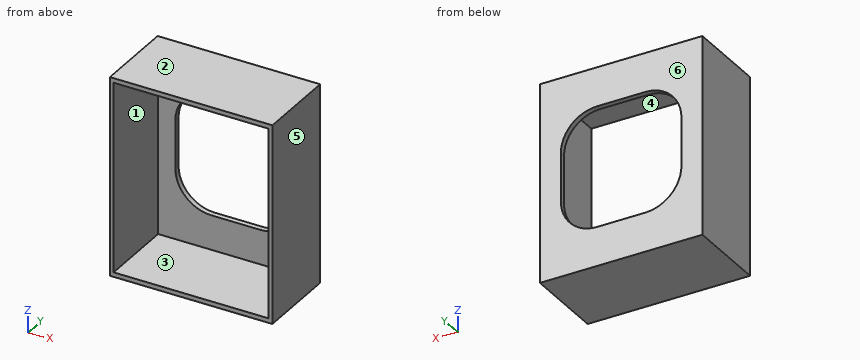
from build123d import *

# Parameters (mm, degrees)
SKETCH1_W           = 90
SKETCH1_H           = 110
BOSS_EXTRUDE1_DEPTH = 3
CUT_EXTRUDE5_DEPTH  = 72.126647608
SKETCH3_W           = 90
SKETCH3_H           = 110
SKETCH3_W_2         = 85.90909091
SKETCH3_H_2         = 105
BOSS_EXTRUDE2_DEPTH = 42


with BuildPart() as part:
    # Sketch1 → Boss-Extrude1 (new body)
    with BuildSketch(Plane(origin=(0, 12.45, 0), x_dir=(1, 0, 0), z_dir=(0, 1, 0))):
        Rectangle(SKETCH1_W, SKETCH1_H)
    extrude(amount=-BOSS_EXTRUDE1_DEPTH)

    # Sketch2 → Cut-Extrude5 (cut, through all)
    with BuildSketch(Plane(origin=(0, 12.45, 0), x_dir=(1, 0, 0), z_dir=(0, 1, 0))):
        with BuildLine():
            Line((-13.4, 33.399999142), (13.4, 33.399999142))
            ThreePointArc((13.4, 33.399999142), (27.542135624, 27.542134765), (33.4, 13.399999142))
            Line((33.4, 13.399999142), (33.4, -13.399999142))
            ThreePointArc((33.4, -13.399999142), (27.542135624, -27.542134765), (13.4, -33.399999142))
            Line((13.4, -33.399999142), (-13.4, -33.399999142))
            ThreePointArc((-13.4, -33.399999142), (-27.542135624, -27.542134765), (-33.4, -13.399999142))
            Line((-33.4, -13.399999142), (-33.4, 13.399999142))
            ThreePointArc((-33.4, 13.399999142), (-27.542135624, 27.542134765), (-13.4, 33.399999142))
        make_face()
    extrude(amount=-CUT_EXTRUDE5_DEPTH, mode=Mode.SUBTRACT)

    # Sketch3 → Boss-Extrude2 (add)
    with BuildSketch(Plane.XZ.offset(-9.45)):
        Rectangle(SKETCH3_W, SKETCH3_H)
        Rectangle(SKETCH3_W_2, SKETCH3_H_2, mode=Mode.SUBTRACT)
    extrude(amount=BOSS_EXTRUDE2_DEPTH)


solid = part.part
Design review of the part built by this model. Coordinates are the model's own, in mm. Face numbers are marked on the shaded views. A direction names the side the tool comes from. Round coordinates to 2 decimals unless told otherwise and drop trailing zeros. Write each loop counter-clockwise with the first axis right and the second up, starting at its lowest first coordinate (ties: lowest second). Pieces come first, ordered by that corner, then holes.
Item 1: For the marked faces 1 and 2, list the 3-axis set-ups (+Z, -Z, +X, -X, +Y, -Y) from which the entire face can be reached by the end or side of a thin tool; tool diameter is ignored.
Item 2: For pin 1 Ø6 at (x, z) = (-33, -20.5) entering from -Y, flat-tipped, find the tip position at first contact; note if it passes through.
Item 3: Wall thickness on L1, parallel to Z at x = 8, y = -9.5; L2, parallel to X at y = -30, z = 47.5; L3, parallel to Y at x = 40.5, z = 13: over which ranges is each line inside the solid? List them lowest first.
Item 4: Consider section D-D on x = 37.5. Give the boundary of the cut face in (y, z), and give its area (3 significant figures).
Item 5: Consider section A-A on x = -19. Give the boundary of the cut face in (y, z), and give its area (3 significant figures).
Item 6: Draft analysis for pull direction X (two halves, no side actions). For the marked faces 3, 4, 5 and 6, state which applies: released by +X, released by -X, zero draft, split by the parting line, or undercut.
Item 7: Consider section C-C on y = -16. Give the boundary of the cut face in (x, z).
Item 8: Consider section B-B on z = -7.5. Give the boundary of the cut face in (x, y).
Check values:
1. face 1: -Y
1. face 2: +Z, +X, -X, +Y, -Y
2. pin 1: stops at y = 9.45
3. L1: z = -55 to -52.5, 52.5 to 55
3. L2: x = -45 to -42.95, 42.95 to 45
3. L3: y = 9.45 to 12.45
4. outline: (-32.55, -55) - (12.45, -55) - (12.45, 55) - (-32.55, 55) - (-32.55, 52.5) - (9.45, 52.5) - (9.45, -52.5) - (-32.55, -52.5) - close
4. area: 540 mm2
5. outline: (-32.55, -55) - (12.45, -55) - (12.45, -32.6) - (9.45, -32.6) - (9.45, -52.5) - (-32.55, -52.5) - close; (-32.55, 52.5) - (9.45, 52.5) - (9.45, 32.6) - (12.45, 32.6) - (12.45, 55) - (-32.55, 55) - close
5. area: 344 mm2
6. face 3: undercut
6. face 4: undercut
6. face 5: released by +X
6. face 6: zero draft
7. outline: (-45, -55) - (45, -55) - (45, 55) - (-45, 55) - close; hole (-42.95, -52.5) - (42.95, -52.5) - (42.95, 52.5) - (-42.95, 52.5) - close
8. outline: (-45, -32.55) - (-42.95, -32.55) - (-42.95, 9.45) - (-33.4, 9.45) - (-33.4, 12.45) - (-45, 12.45) - close; (33.4, 9.45) - (42.95, 9.45) - (42.95, -32.55) - (45, -32.55) - (45, 12.45) - (33.4, 12.45) - close
